from build123d import *

# Parameters (mm, degrees)
SKETCH2_R           = 7.5
BOSS_EXTRUDE1_DEPTH = 5
SKETCH2_3_R         = 12
SKETCH2_3_R_2       = 7.5
BOSS_EXTRUDE2_DEPTH = 2
BOSS_EXTRUDE4_START = -2
SKETCH2_5_R         = 7.5
BOSS_EXTRUDE4_DEPTH = 2
SKETCH4_R           = 7.5
BOSS_EXTRUDE5_DEPTH = 5
CUT_EXTRUDE1_DEPTH  = 21.784609691


with BuildPart() as part:
    # Sketch2 → Boss-Extrude1 (new body)
    with BuildSketch(Plane(origin=(0, 0, 0), x_dir=(1, 0, 0), z_dir=(0, 1, 0))):
        with Locations(Location((0, 0, 0), (0, 0, 270))):
            Circle(SKETCH2_R)
    extrude(amount=BOSS_EXTRUDE1_DEPTH)



with BuildPart() as body_2:
    # Sketch2_3 → Boss-Extrude2 (new body)
    with BuildSketch(Plane(origin=(0, 0, 0), x_dir=(1, 0, 0), z_dir=(0, 1, 0))):
        with Locations(Location((0, 0, 0), (0, 0, 270))):
            Circle(SKETCH2_3_R)
        with Locations(Location((0, 0, 0), (0, 0, 270))):
            Circle(SKETCH2_3_R_2, mode=Mode.SUBTRACT)
    extrude(amount=-BOSS_EXTRUDE2_DEPTH)


with BuildPart() as part_1:
    add(part.part)

    add(body_2.part)  # Boss-Extrude4 merges body 2
    # Sketch2_5 → Boss-Extrude4 (add)
    with BuildSketch(Plane(origin=(0, 0, 0), x_dir=(1, 0, 0), z_dir=(0, 1, 0)).offset(BOSS_EXTRUDE4_START)):
        with Locations(Location((0, 0, 0), (0, 0, 270))):
            Circle(SKETCH2_5_R)
    extrude(amount=BOSS_EXTRUDE4_DEPTH)

    # Sketch4 → Boss-Extrude5 (add)
    with BuildSketch(Plane.XZ.offset(2)):
        with Locations(Location((3, 0, 0), (0, 0, 270))):
            Circle(SKETCH4_R)
    extrude(amount=BOSS_EXTRUDE5_DEPTH)

    # Sketch6 → Cut-Extrude1 (cut, through all)
    with BuildSketch(Plane(origin=(0, 5, 0), x_dir=(1, 0, 0), z_dir=(0, 1, 0))):
        with BuildLine():
            Line((-0.85, -1.112429773), (-0.85, 1.112429773))
            ThreePointArc((-0.85, 1.112429773), (4.1, 0), (-0.85, -1.112429773))
        make_face()
    extrude(amount=-CUT_EXTRUDE1_DEPTH, mode=Mode.SUBTRACT)


solid = part_1.part
The listing builds one solid part. Answer for the finished solid, in the listing's coordinates (mm). A direction names the side the tool comes from. Coordinates: 2 decimals unless noted, no trailing zeros. Loops run counter-clockwise (first coordinate to the right, second up) from the corner with the lowest first, then second, coordinate; pieces in that order, holes last.
1) Determine the mould class of faces 1 (the face through (3.604, -0.986, 11.446)), 2 (the face through (-5, 0, -6)), 3 (the face through (-0.85, -1, 0)) for opening direction Z: pulls with the +Z half, pulls with the -Z half, needs draft (parallel to the pull), parting line crosses it, or undercut.
2) Find the intervals of material crossed by L1, parallel to X at y = -0.5, z = 0; L2, parallel to X at y = -2.75, z = 0; L3, parallel to Z at x = 1.5, y = 2, in increasing order.
3) Find section B-B on x = 0. Write down the section's boundary in (y, z).
4) A tool of negligible diameter and unlimited length cuts with its end or side. For faces 4 (the face through (-2, 5, 0)), 5 (the face through (0.33, 2.465, -7.493)), 6 (the face through (10.436, -4.465, 0.976)), from which of +Z, -Z, +X, -X, +Y, -Y can it reach the whole face along a straight path? Write none if from no direction.
5) Flat-ended cylindrical pins translate along their axes: pin 1 Ø3 at (x, z) = (8.5, -6.5) entering from +Y; pin 2 Ø3 at (x, y) = (-4.5, -1) entering from -Z; pin 3 Ø6 at (x, y) = (9.5, 0.5) entering from +Z; pin 4 Ø3 at (x, z) = (1.5, 0) entering from -Y. Find the tip coordinate at first contact, or state that the pin passes through.
6) Find section C-C on y = 2.75. Write down the section's boundary in (x, z), then the cut area to 3 significant figures.
7) Find section D-D on x = 9.25. Write down the section's boundary in (y, z).
8) Find section A-A on z = 0. Write down the section's boundary in (x, y).
Values:
1. face 1: parting line crosses it
1. face 2: needs draft
1. face 3: undercut
2. L1: x = -12 to -0.85, 4.1 to 12
2. L2: x = -4.5 to -0.85, 4.1 to 10.5
2. L3: z = -7.35 to -2.6, 2.6 to 7.35
3. outline: (-7, -6.87) - (-2, -6.87) - (-2, -12) - (0, -12) - (0, -7.5) - (5, -7.5) - (5, -2.12) - (-7, -2.12) - close; (-7, 2.12) - (5, 2.12) - (5, 7.5) - (0, 7.5) - (0, 12) - (-2, 12) - (-2, 6.87) - (-7, 6.87) - close
4. face 4: +Z, -Z, +X, -X, +Y
4. face 5: +Y
4. face 6: -Y
5. pin 1: stops at y = 0
5. pin 2: stops at z = -11.62
5. pin 3: stops at z = 10.06
5. pin 4: passes through
6. outline: circle Ø15 at (0, 0); hole (-0.85, -1.11) arc R2.6 ccw (long way) to (-0.85, 1.11) - close
6. area: 156 mm2
7. outline: (-7, -4.15) - (-2, -4.15) - (-2, -7.64) - (0, -7.64) - (0, 7.64) - (-2, 7.64) - (-2, 4.15) - (-7, 4.15) - close
8. outline: (-12, -2) - (-4.5, -2) - (-4.5, -7) - (-0.85, -7) - (-0.85, 5) - (-7.5, 5) - (-7.5, 0) - (-12, 0) - close; (4.1, -7) - (10.5, -7) - (10.5, -2) - (12, -2) - (12, 0) - (7.5, 0) - (7.5, 5) - (4.1, 5) - close
